Verification items for the finished model (mm, model axes). A direction names the side the tool comes from. Give positions to 0.01 mm unless a question says otherwise; leave off trailing zeros. Order: outer loops, then holes, each group sorted by start corner. A loop starts at its lowest first (then second) coordinate and runs counter-clockwise, first axis right, second up.
from build123d import *

# Parameters (mm, degrees)
F3_R     = 1.75
F4_DEPTH = 6
F5_R     = 3.25
F6_DEPTH = 3


with BuildPart() as f1:
    # F0 (on Top) → F1 (revolve)
    with BuildSketch(Plane.XY):
        with BuildLine():
            Line((-3, 0), (3, 0))
            Line((3, 0), (3, 10))
            Line((3, 10), (1.5, 10))
            ThreePointArc((1.5, 10), (0, 8.5), (-1.5, 10))
            Line((-1.5, 10), (-3, 10))
            Line((-3, 10), (-3, 0))
        make_face()
    revolve(axis=Axis((0, 0, 0), (1, 0, 0)))

    # F3 (on offset) → F4 (cut, through all)
    with BuildSketch(Plane(origin=(-3, 0, 0), x_dir=(0, -1, 0), z_dir=(-1, 0, 0))):
        Circle(F3_R)
    extrude(amount=-F4_DEPTH, mode=Mode.SUBTRACT)

    # F5 (on offset) → F6 (cut)
    with BuildSketch(Plane(origin=(-3, 0, 0), x_dir=(0, -1, 0), z_dir=(-1, 0, 0))):
        Circle(F5_R)
    extrude(amount=-F6_DEPTH, mode=Mode.SUBTRACT)


solid = f1.part
(1) Section check A-A, the plane z = 0. Enter the section's corners in (x, y).
Solved:
outline: (-3, -10) - (-1.5, -10) arc R1.5 cw to (1.5, -10) - (3, -10) - (3, -1.75) - (0, -1.75) - (0, -3.25) - (-3, -3.25) - close; (-3, 3.25) - (0, 3.25) - (0, 1.75) - (3, 1.75) - (3, 10) - (1.5, 10) arc R1.5 cw to (-1.5, 10) - (-3, 10) - close
(2) Release check for a two-part mould opening along Y. For faces 1 (the flat face through (3, -2, 0)), 2 (the cylindrical face through (2.24, -2.17, -9.76)), 3 (the flat face through (0, -1.4, -1.4)) record: pulls with the +Y half, pulls with the -Y half, needs draft (parallel to the pull), parting line crosses it, or undercut.
Solved:
face 1: needs draft
face 2: parting line crosses it
face 3: undercut
(3) Set-up check for faces 4 (the flat face through (-3, 4, 0)), 5 (the cylindrical face through (-1.521, 2.579, -1.978)): record each of +Z, -Z, +X, -X, +Y, -Y from which the full face is reachable in a straight line by a thin tool's end or side.
Solved:
face 4: +Z, -Z, -X, +Y, -Y
face 5: -X
(4) Go/stop test with flat-tipped pins: pin 1 (1 mm diameter, centred on x = 0, y = 6.5, fed in from +Z); pin 2 (2 mm diameter, centred on y = -1, z = 0.5, fed in from -X); pin 3 (3 mm diameter, centred on x = -2, y = -4.5, fed in from +Z). Record where each tip stops, or that it passes through.
Solved:
pin 1: stops at z = 6.02
pin 2: stops at x = 0
pin 3: stops at z = 9.54
(5) Scan lines: line 1 (Z direction, x = -2.4, y = 0); line 2 (Z direction, x = -0.7, y = 0); line 3 (X direction, y = -5.75, z = -7.25). Record each from-to range of solid material in increasing order.
Solved:
line 1: z = -10 to -3.25, 3.25 to 10
line 2: z = -8.67 to -3.25, 3.25 to 8.67
line 3: x = -3 to -1.3, 1.3 to 3
(6) Section check D-D, the plane x = -2.1. Enter the section's corners in (y, z).
Solved:
outline: circle Ø20 at (0, 0); hole circle Ø6.5 at (0, 0)
(7) Section check C-C, the plane x = 1.9. Enter the section's corners in (y, z), then the cut area to 3 significant figures.
Solved:
outline: circle Ø20 at (0, 0); hole circle Ø3.5 at (0, 0)
area: 305 mm2
